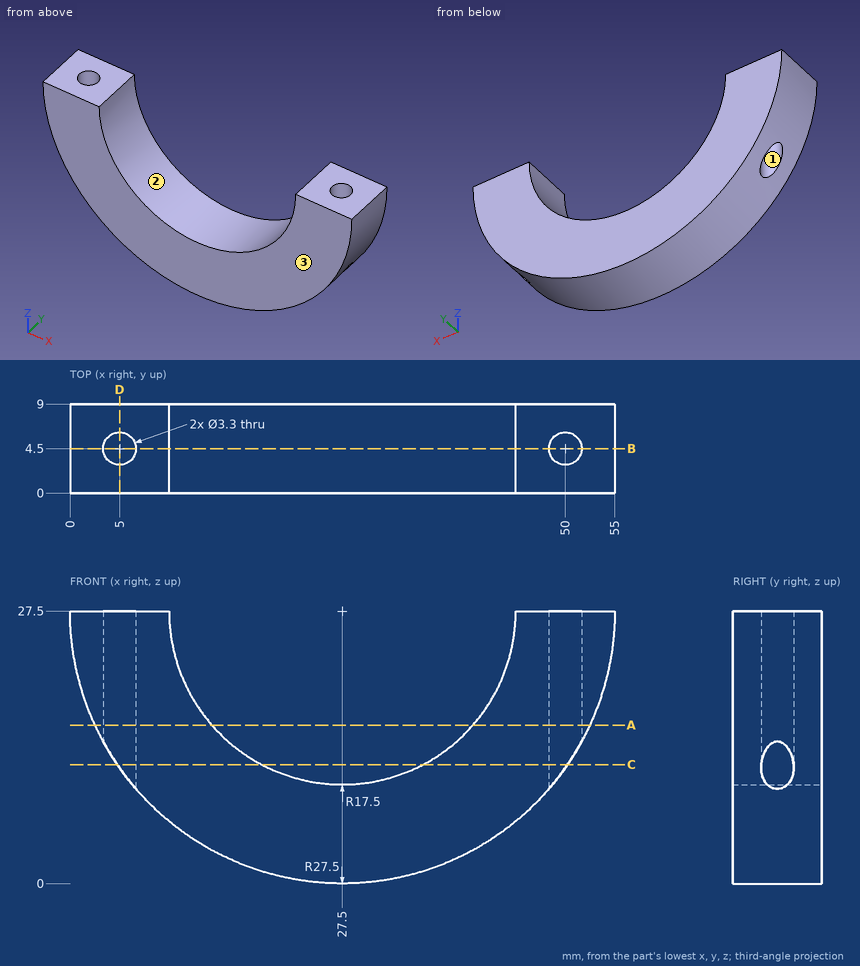
Check sheet for the drawn part. Datum: minimum x, y, z corner. Units: mm. Coordinates: 2 decimals unless noted, no trailing zeros. Loops run counter-clockwise (first coordinate to the right, second up) from the corner with the lowest first, then second, coordinate; pieces in that order, holes last. Notation, with made-up numbers: (-9.75, 45.5) -> (32.25, 45.5) arc R17 cw to (32.25, 74.5) -> close; hole circle Ø6 at (58.5, 12.25). An arc over 180 degrees is marked (long way). Write each question's results on one line, items separated by ' | '.
Item 1: Section check B-B, the plane y = 4.5. Enter the section's corners in (x, z).
Found:
outline: (0, 27.5) arc R27.5 ccw to (3.35, 14.35) -> (3.35, 27.5) -> close; (6.65, 9.57) arc R27.5 ccw to (48.35, 9.57) -> (48.35, 27.5) -> (45, 27.5) arc R17.5 cw to (10, 27.5) -> (6.65, 27.5) -> close; (51.65, 14.35) arc R27.5 ccw to (55, 27.5) -> (51.65, 27.5) -> close
Item 2: Gauge pin test, flat ends, axial feed: pin 1 (4 mm diameter, centred on x = 50, y = 4.5, fed in from -Z); pin 2 (1 mm diameter, centred on y = 3.5, z = 4, fed in from +X); pin 3 (4.5 mm diameter, centred on x = 5, y = 4.5, fed in from -Z). Record the tip position at first contact, or that the pin passes through.
Found:
pin 1: stops at z = 9.17 | pin 2: stops at x = 42.57 | pin 3: stops at z = 8.89
Item 3: Section check A-A, the plane z = 16. Enter the section's corners in (x, y).
Found:
outline: (2.52, 0) -> (14.31, 0) -> (14.31, 9) -> (2.52, 9) -> close; (40.69, 0) -> (52.48, 0) -> (52.48, 9) -> (40.69, 9) -> close; hole circle Ø3.3 at (5, 4.5); hole circle Ø3.3 at (50, 4.5)
Item 4: Mould release check, pull along Y, two halves, no side actions. Record for the marked faces 1, 2 and 3: +Y half, -Y half, draft (parallel to the pull), parting line (faces both ways), or undercut.
Found:
face 1: undercut | face 2: draft | face 3: -Y half
Item 5: Material ranges on L1, parallel to Y at x = 5, z = 17.75; L2, parallel to X at y = 5.25, z = 16; L3, parallel to X at y = 5, z = 16.25, recorded low to high.
Found:
L1: y = 0 to 2.85, 6.15 to 9 | L2: x = 2.52 to 3.53, 6.47 to 14.31, 40.69 to 48.53, 51.47 to 52.48 | L3: x = 2.41 to 3.43, 6.57 to 14.1, 40.9 to 48.43, 51.57 to 52.59
Item 6: Section check D-D, the plane x = 5. Enter the section's corners in (y, z), plus the area to 3 significant figures.
Found:
outline: (0, 11.69) -> (2.85, 11.69) -> (2.85, 27.5) -> (0, 27.5) -> close; (6.15, 11.69) -> (9, 11.69) -> (9, 27.5) -> (6.15, 27.5) -> close | area: 90.1 mm2
Item 7: Section check C-C, the plane z = 12. Enter the section's corners in (x, y).
Found:
outline: (4.78, 0) -> (19.38, 0) -> (19.38, 9) -> (4.78, 9) -> (4.78, 6.14) arc R1.65 cw (long way) to (4.78, 2.86) -> close; (35.62, 0) -> (50.22, 0) -> (50.22, 2.86) arc R1.65 cw (long way) to (50.22, 6.14) -> (50.22, 9) -> (35.62, 9) -> close
